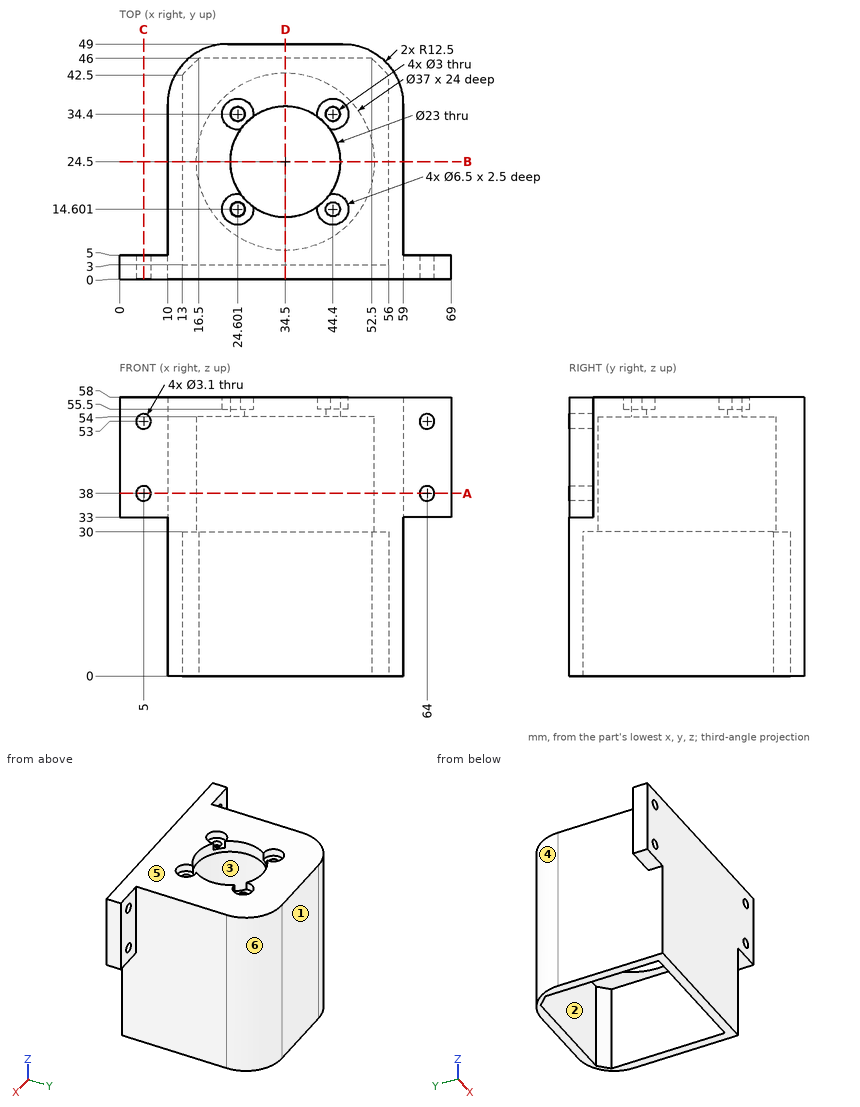
Here's the drawing with two shaded views (mm, measured from the low corner). I have some questions. A direction names the side the tool comes from. Coordinates: 2 decimals unless noted, no trailing zeros. Write each loop counter-clockwise with the first axis right and the second up, starting at its lowest first coordinate (ties: lowest second). Pieces come first, ordered by that corner, then holes. Notation, with made-up numbers: M 70.5,69 L 119.5,69 A24 ccw 119.5,107 Z; hole C 47.5,-17.75 d5. An arc over 180 degrees is marked long. Write item = value, one per line. Start each with the question number.
Q1. On a 3-axis mill with a long thin cutter (end or side, diameter ignored), from which of +Z, -Z, +X, -X, +Y, -Y can I reach the whole of each face in a straight line? I mean the marked faces 1 and 2. Say none if no direction works.
Q2. I'm going to push flat-ended pins straight in: pin 1 (8 mm diameter, centred on y = 18.5, z = 15, fed in from -X); pin 2 (8.5 mm diameter, centred on x = 24.6, y = 14.6, fed in from -Z); pin 3 (5 mm diameter, centred on x = 61.5, y = 43, fed in from +Z); pin 4 (5 mm diameter, centred on x = 63.5, z = 51, fed in from +Y). Where does each tip first touch, or does it pass through?
Q3. If we section it at B-B, the plane y = 24.5: Write out the boundary of the cut face in (x, z), then the cut area to 3 significant figures.
Q4. If we section it at D-D, the plane x = 34.5: Write out the boundary of the cut face in (y, z).
Q5. If we section it at C-C, the plane x = 5: Write out the boundary of the cut face in (y, z).
Q6. If I drill on L1, parallel to Z at x = 64, y = 3.55; L2, parallel to Y at x = 38, z = 16.5; L3, parallel to Y at x = 34, z = 36, over which ranges is the centre line in solid material (lowest first)? Write a range as [from, to].
Q7. If we section it at A-A, the plane z = 38: Write out the boundary of the cut face in (x, y).
Q8. Thinking about a two-plate mould opening in X: for the marked faces 3, 4, 5 and 6, which applies, released by +X, released by -X, zero draft, split by the parting line, or undercut?
Check sheet entries:
q1.face_1 = +Z, -Z, +X, -X, +Y
q1.face_2 = -Z
q2.pin_1 = 10
q2.pin_2 = 54
q2.pin_3 = through
q2.pin_4 = 5
q3.outline = M 10,0 L 13,0 L 13,30 L 16,30 L 16,54 L 23,54 L 23,58 L 10,58 Z; M 46,54 L 53,54 L 53,30 L 56,30 L 56,0 L 59,0 L 59,58 L 46,58 Z
q3.area = 572 mm²
q4.outline = M 0,0 L 3,0 L 3,30 L 6,30 L 6,54 L 13,54 L 13,58 L 0,58 Z; M 36,54 L 43,54 L 43,30 L 46,30 L 46,0 L 49,0 L 49,58 L 36,58 Z
q5.outline = M 0,33 L 5,33 L 5,36.45 L 0,36.45 Z; M 0,39.55 L 5,39.55 L 5,51.45 L 0,51.45 Z; M 0,54.55 L 5,54.55 L 5,58 L 0,58 Z
q6.L1 = [33, 36.45], [39.55, 51.45], [54.55, 58]
q6.L2 = [0, 3], [46, 49]
q6.L3 = [0, 6.01], [42.99, 49]
q7.outline = M 0,0 L 3.45,0 L 3.45,5 L 0,5 Z; M 6.55,0 L 62.45,0 L 62.45,5 L 59,5 L 59,36.5 A12.5 ccw 46.5,49 L 22.5,49 A12.5 ccw 10,36.5 L 10,5 L 6.55,5 Z; M 65.55,0 L 69,0 L 69,5 L 65.55,5 Z; hole C 34.5,24.5 d37
q8.face_3 = undercut
q8.face_4 = released by -X
q8.face_5 = zero draft
q8.face_6 = released by +X
